For this review, use the dimensioned drawing (mm, ordinates from the lowest corner) and the shaded views. A direction names the side the tool comes from. Coordinates: 2 decimals unless noted, no trailing zeros. Loops run counter-clockwise (first coordinate to the right, second up) from the corner with the lowest first, then second, coordinate; pieces in that order, holes last. Notation, with made-up numbers: (-39.5, -17) - (-2.5, -17) arc R22 cw to (-2.5, 14) - close; hole circle Ø6 at (62.25, -26.5). An arc over 180 degrees is marked (long way). Return JSON: item names as keys, results as strings. Group by question number.
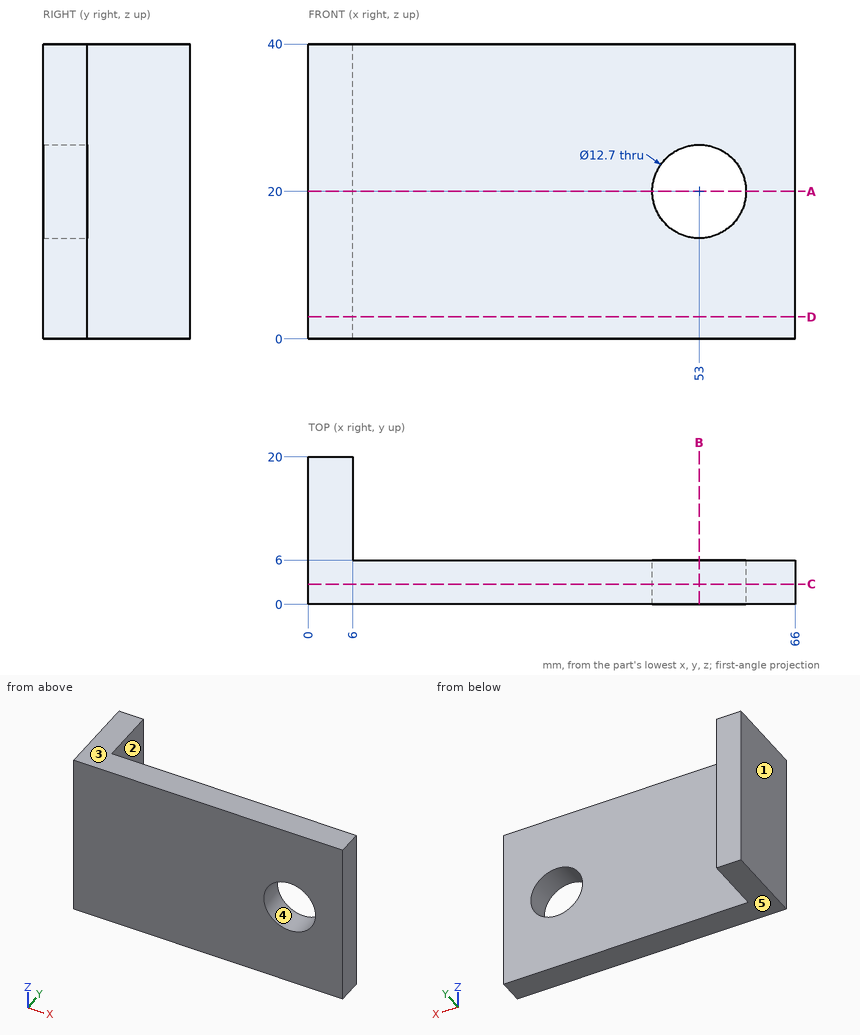
Item 1: Add section D-D (z = 3). State the section outline as (x, y) points.
Item 2: Add section A-A (z = 20). State the section outline as (x, y) points.
Item 3: Add section C-C (y = 2.75). State the section outline as (x, z) points.
Item 4: For the marked faces 1 and 2, list the 3-axis set-ups (+Z, -Z, +X, -X, +Y, -Y) from which the entire face can be reached by the end or side of a thin tool; tool diameter is ignored.
Item 5: Draft analysis for pull direction Z (two halves, no side actions). For the marked faces 3, 4 and 5, state which applies: pulls with the +Z half, pulls with the -Z half, needs draft (parallel to the pull), parting line crosses it, or undercut.
Item 6: Add section B-B (x = 53). State the section outline as (y, z) points, then the cut area to 3 significant figures.
Item 7: To check wall thickness, follow line 1 (Z direction, x = 53, y = 2.3); line 2 (X direction, y = 4.65, z = 20); line 3 (X direction, y = 14, z = 27). State the ranges of each line that lie inside material, in increasing order. Write a range as from..to.
Item 8: For P1, Ø20, axis at x = 27.5, z = 19.5, coming from the +Y side; P2, Ø5, axis at x = 8, z = 11.5, coming from the -Y side; P3, Ø4, axis at y = 14, z = 27, coming from the +X side, all flat-tipped, find the tip position at first contact; note any pin that passes through.
Answers below:
{
 "1": {"outline": "(0, 0) - (66, 0) - (66, 6) - (6, 6) - (6, 20) - (0, 20) - close"},
 "2": {"outline": "(0, 0) - (46.65, 0) - (46.65, 6) - (6, 6) - (6, 20) - (0, 20) - close; (59.35, 0) - (66, 0) - (66, 6) - (59.35, 6) - close"},
 "3": {"outline": "(0, 0) - (66, 0) - (66, 40) - (0, 40) - close; hole circle Ø12.7 at (53, 20)"},
 "4": {"face 1": "+Z, -Z, -X, +Y, -Y", "face 2": "+Z, -Z, +X, +Y"},
 "5": {"face 3": "pulls with the +Z half", "face 4": "undercut", "face 5": "pulls with the -Z half"},
 "6": {"outline": "(0, 0) - (6, 0) - (6, 13.65) - (0, 13.65) - close; (0, 26.35) - (6, 26.35) - (6, 40) - (0, 40) - close", "area": "164 mm^2"},
 "7": {"line 1": "z = 0..13.65, 26.35..40", "line 2": "x = 0..46.65, 59.35..66", "line 3": "x = 0..6"},
 "8": {"P1": "stops at y = 6", "P2": "stops at y = 0", "P3": "stops at x = 6"}
}
